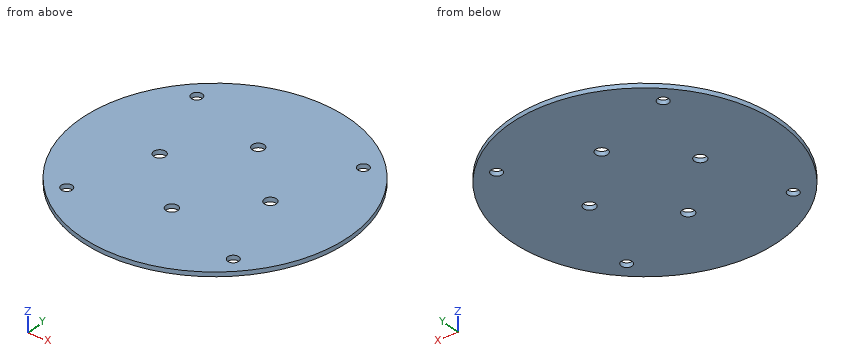
```python
from build123d import *

# Parameters (mm, degrees)
SKETCH3_R                       = 49
BOSS_EXTRUDE1_DEPTH             = 1.6
F_4_0MM_CLEARANCE_DOWEL_HOLE1_D = 4
SKETCH7_R                       = 2.183129746
CUT_EXTRUDE1_DEPTH              = 70.314933456


with BuildPart() as part:
    # Sketch3 → Boss-Extrude1 (new body)
    with BuildSketch(Plane.XY):
        Circle(SKETCH3_R)
    extrude(amount=BOSS_EXTRUDE1_DEPTH)

    # Ø4.0mm Clearance Dowel Hole1 (through all)
    with Locations(Plane(origin=(0, 0, 0), x_dir=(1, 0, 0), z_dir=(0, 0, -1))):
        with Locations((-30.087393539, -30.08739354), (30.087393539, -30.08739354), (30.087393539, 30.087393539), (-30.08739354, 30.087393539)):
            Hole(F_4_0MM_CLEARANCE_DOWEL_HOLE1_D / 2)

    # Sketch7 → Cut-Extrude1 (cut, through all)
    with BuildSketch(Plane.XY):
        with Locations((0, 20)):
            Circle(SKETCH7_R)
        with Locations((20, 0)):
            Circle(SKETCH7_R)
        with Locations((0, -20)):
            Circle(SKETCH7_R)
        with Locations((-20, 0)):
            Circle(SKETCH7_R)
    extrude(amount=CUT_EXTRUDE1_DEPTH, mode=Mode.SUBTRACT)


solid = part.part
```
Design review of the part built by this model. Coordinates are the model's own, in mm. Round coordinates to 2 decimals unless told otherwise and drop trailing zeros. Write each loop counter-clockwise with the first axis right and the second up, starting at its lowest first coordinate (ties: lowest second). Pieces come first, ordered by that corner, then holes. Notation, with made-up numbers: (-33.5, -30.5) -> (3.5, -30.5) arc R35 ccw to (3.5, 7.5) -> close; hole circle Ø10 at (64, -21). An arc over 180 degrees is marked (long way). Answer in a Markdown table with one row per item.
Q1. Clearance check with a flat-ended pin moving along its axis: pin 1 Ø2.5 at (x, y) = (30.09, 30.09) entering from +Z. State where the tip first meets the part, or that it passes through.
The answers:
| item | result |
|---|---|
| pin 1 | through |
Q2. Take a section at D-D, the plane z = 0.25. Count the separate pieces of the cut face and the enclosed holes in it, then the cut area to 3 significant figures.
The answers:
| item | result |
|---|---|
| separate pieces | 1 |
| enclosed holes | 8 |
| area | 7,430 mm² |
Q3. Take a section at C-C, the plane x = 20. State the section outline as (y, z) points.
The answers:
| item | result |
|---|---|
| outline | (-44.73, 0) -> (-2.18, 0) -> (-2.18, 1.6) -> (-44.73, 1.6) -> close; (2.18, 0) -> (44.73, 0) -> (44.73, 1.6) -> (2.18, 1.6) -> close |
Q4. Take a section at A-A, the plane x = 0. State the section outline as (y, z) points, then the cut area to 3 significant figures.
The answers:
| item | result |
|---|---|
| outline | (-49, 0) -> (-22.18, 0) -> (-22.18, 1.6) -> (-49, 1.6) -> close; (-17.82, 0) -> (17.82, 0) -> (17.82, 1.6) -> (-17.82, 1.6) -> close; (22.18, 0) -> (49, 0) -> (49, 1.6) -> (22.18, 1.6) -> close |
| area | 143 mm² |
Q5. To check wall thickness, follow L1, parallel to Y at x = 0, z = 0.55; L2, parallel to Y at x = 20, z = 0.4; L3, parallel to X at y = 1, z = 0.8. State the ranges of each line that lie inside material, in increasing order. Write a range as [from, to].
The answers:
| item | result |
|---|---|
| L1 | [-49, -22.18], [-17.82, 17.82], [22.18, 49] |
| L2 | [-44.73, -2.18], [2.18, 44.73] |
| L3 | [-48.99, -21.94], [-18.06, 18.06], [21.94, 48.99] |
